The drawing under review shows one solid part. Ordinate dimensions are in mm from its lowest x, y, z. Round coordinates to 2 decimals unless told otherwise and drop trailing zeros. Order: outer loops, then holes, each group sorted by start corner. A loop starts at its lowest first (then second) coordinate and runs counter-clockwise, first axis right, second up. Notation, with made-up numbers: M 56.25,51 L 106.25,51 A34 cw 106.25,89 Z; hole C 88,-13.75 d10. An arc over 180 degrees is marked long. Answer in a Markdown table with one row per item. Add a question column.
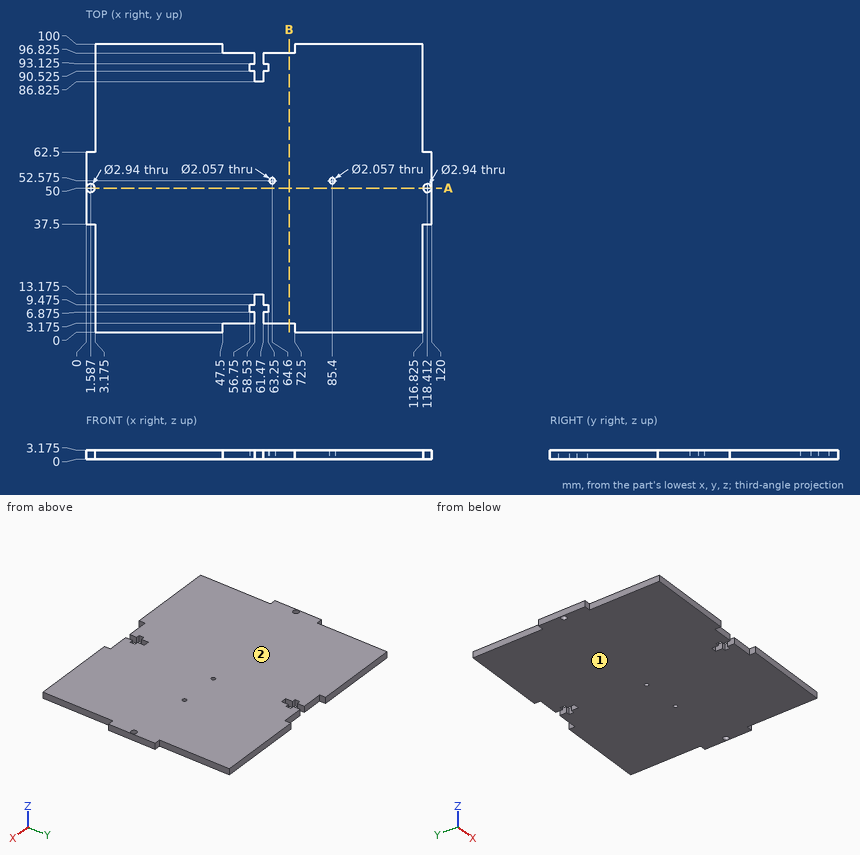
1. The part is to be moulded in two halves that separate along Z. For the marked faces 1 and 2, say which applies: pulls with the +Z half, pulls with the -Z half, needs draft (parallel to the pull), parting line crosses it, or undercut.
2. To check wall thickness, follow probe 1 along X at (y, z) = (90, 1.05) (1 decimal); probe 2 along Y at (x, z) = (85.4, 1); probe 3 along X at (y, z) = (66, 1.55) (1 decimal). State the ranges of each line that lie inside material, in increasing order. Write a range as [from, to].
3. Consider section A-A on y = 50. State how many separate pieces and enclosed holes the cut face has.
4. Consider section B-B on x = 70.5. Write out the cut boundary in (y, z) (1 decimal).
5. Clearance check with flat-ended pins moving along their axes: pin 1 Ø1.4 at (x, z) = (58, 2) entering from +Y (1 decimal); pin 2 Ø1.8 at (x, y) = (1.59, 50) entering from +Z; pin 3 Ø1 at (x, z) = (1, 1) entering from -Y; pin 4 Ø1 at (y, z) = (89.5, 1.5) entering from -X (1 decimal). State where each tip first meets the part, or that it passes through.
Solved:
| question | item | result |
|---|---|---|
| 1 | face 1 | pulls with the -Z half |
| 1 | face 2 | pulls with the +Z half |
| 2 | probe 1 | x = [3.2, 58.5], [61.5, 116.8] |
| 2 | probe 2 | y = [0, 51.55], [53.6, 100] |
| 2 | probe 3 | x = [3.2, 116.8] |
| 3 | separate pieces | 3 |
| 3 | enclosed holes | 0 |
| 4 | outline | M 3.2,0 L 96.8,0 L 96.8,3.2 L 3.2,3.2 Z |
| 5 | pin 1 | stops at y = 96.8 |
| 5 | pin 2 | passes through |
| 5 | pin 3 | stops at y = 37.5 |
| 5 | pin 4 | stops at x = 3.2 |
